from build123d import *

# Parameters (mm, degrees)
REDONDEO2_R = 2
REDONDEO3_R = 0.5


with BuildPart() as part:
    # Croquis1 → Revolución1 (revolve)
    with BuildSketch(Plane.XY, mode=Mode.PRIVATE) as revoluci_n1_sk:
        Polygon((-16, 2.5), (-16, 30), (-11, 30), (-6.179413414, 16), (0, 16), (0, 2.5), align=None)
    revolve(revoluci_n1_sk.sketch.rotate(Axis((-29.031578947, 0, 0), (1, 0, 0)), 90), axis=Axis((-29.031578947, 0, 0), (1, 0, 0)))

    # Redondeo2
    redondeo2_edges = [part.edges().sort_by_distance(p)[0] for p in [
        (-16, 0, -30),
    ]]
    fillet(redondeo2_edges, radius=REDONDEO2_R)

    # Redondeo3
    redondeo3_edges = [part.edges().sort_by_distance(p)[0] for p in [
        (-16, 0, -2.5),
    ]]
    fillet(redondeo3_edges, radius=REDONDEO3_R)

    # Simetría2: part across plane


with BuildPart() as part_1:
    add(part.part)
    add(part.part.mirror(Plane(origin=(0, 0, 0), x_dir=(0, 0, 1), z_dir=(1, 0, 0))))


solid = part_1.part
CAD build for the part. Positions are in the model's coordinates, mm. A direction names the side the tool comes from. Coordinates: 2 decimals unless noted, no trailing zeros. Loops run counter-clockwise (first coordinate to the right, second up) from the corner with the lowest first, then second, coordinate; pieces in that order, holes last. Notation, with made-up numbers: (-32.5, 1.25) -> (16.5, 1.25) arc R14 ccw to (16.5, 7.25) -> close; hole circle Ø4 at (68, 17). An arc over 180 degrees is marked (long way). One line per item, written item: value.
1. Slice it at D-D on x = -13. Write the cut outline in (y, z).
Answers:
outline: circle Ø60 at (0, 0); hole circle Ø5 at (0, 0)
2. Drill centre lines: line 1 (Y direction, x = -5, z = 0); line 2 (X direction, y = 15, z = 19); line 3 (X direction, y = -17.5, z = 22.5). Where is each one in solid material? Low to high. Write a range as [from, to].
Answers:
line 1: y = [-16, -2.5], [2.5, 16]
line 2: x = [-16, -9.01], [9.01, 16]
line 3: x = [-15.94, -10.49], [10.49, 15.94]
3. Slice it at A-A on y = 0. Write the cut outline in (x, z), and give its area (3 significant figures).
Answers:
outline: (-16, -28) arc R2 ccw to (-14, -30) -> (-11, -30) -> (-6.18, -16) -> (6.18, -16) -> (11, -30) -> (14, -30) arc R2 ccw to (16, -28) -> (16, -3) arc R0.5 ccw to (15.5, -2.5) -> (-15.5, -2.5) arc R0.5 ccw to (-16, -3) -> close; (-16, 3) arc R0.5 ccw to (-15.5, 2.5) -> (15.5, 2.5) arc R0.5 ccw to (16, 3) -> (16, 28) arc R2 ccw to (14, 30) -> (11, 30) -> (6.18, 16) -> (-6.18, 16) -> (-11, 30) -> (-14, 30) arc R2 ccw to (-16, 28) -> close
area: 1,280 mm^2
4. Pull direction X, two halves, no side cores. Call faces 3 (the face through (12.479, -25.296, 16.128)), 4 (the face through (6.4, -16.5, -2.2)), 5 (the face through (16, 6, 0)): pulls with the +X half, pulls with the -X half, needs draft (parallel to the pull), parting line crosses it, or undercut.
Answers:
face 3: needs draft
face 4: undercut
face 5: pulls with the +X half
5. Flat gauge pins, fed straight in: P1, Ø10, axis at x = 1.5, y = 13.5, coming from the +Z side; P2, Ø3, axis at y = 23.5, z = -23, coming from the -X side; P3, Ø2, axis at x = -4, z = 2.5, coming from the -Y side; P4, Ø4, axis at x = -2.5, y = 0.5, coming from the +Z side. Where does each tip first touch, or does it go through?
Answers:
P1: stops at z = 13.56
P2: passes through
P3: stops at y = -15.93
P4: stops at z = 16
6. Which spindle directions (+Z, -Z, +X, -X, +Y, -Y) get a long thin tool onto all of the face, cutting with end or side? Do faces 1 (the face through (-6.4, -16.5, -2.2)), 2 (the face through (-16, 6, 0)). Say none if no direction does.
Answers:
face 1: none
face 2: +Z, -Z, -X, +Y, -Y
7. Slice it at C-C on x = -4.5. Write the cut outline in (y, z), and give its area (3 significant figures).
Answers:
outline: circle Ø32 at (0, 0); hole circle Ø5 at (0, 0)
area: 785 mm^2
